Part model, mm, in its own coordinate system. Coordinates: 2 decimals unless noted, no trailing zeros. Order: outer loops, then holes, each group sorted by start corner. A loop starts at its lowest first (then second) coordinate and runs counter-clockwise, first axis right, second up.
from build123d import *

# Parameters (mm, degrees)
SKETCH019_W     = 73
SKETCH019_H     = 40
PAD006_DEPTH    = 5
SKETCH020_R     = 3
SKETCH020_R_2   = 1.75
POCKET011_DEPTH = 5
SKETCH021_R     = 3
POCKET012_DEPTH = 3.5
FILLET_R        = 1
POCKET014_DEPTH = 1


with BuildPart() as part:
    # Sketch019 → Pad006 (new body)
    with BuildSketch(Plane.XY):
        with Locations((36.5, 20)):
            Rectangle(SKETCH019_W, SKETCH019_H)
    extrude(amount=PAD006_DEPTH)

    # Sketch020 (on Face6 of Pad006) → Pocket011 (cut)
    with BuildSketch(Plane.XY.offset(5)):
        with Locations((14, 18.5)):
            Circle(SKETCH020_R)
        with Locations((59, 18.5)):
            Circle(SKETCH020_R)
        with Locations((36.5, 18.5)):
            Circle(SKETCH020_R)
        with Locations((9, 33.25)):
            Circle(SKETCH020_R_2)
        with Locations((64, 33.25)):
            Circle(SKETCH020_R_2)
        with Locations((64, 5.25)):
            Circle(SKETCH020_R_2)
        with Locations((9, 5.25)):
            Circle(SKETCH020_R_2)
    extrude(amount=-POCKET011_DEPTH, mode=Mode.SUBTRACT)

    # Sketch021 (on Face5 of Pocket011) → Pocket012 (cut)
    with BuildSketch(Plane.XY.offset(5)):
        with Locations((36.5, 18.5)):
            Circle(SKETCH021_R)
        with Locations((9, 5.25)):
            Circle(SKETCH021_R)
        with Locations((64, 33.25)):
            Circle(SKETCH021_R)
        with Locations((9, 33.25)):
            Circle(SKETCH021_R)
    extrude(amount=-POCKET012_DEPTH, mode=Mode.SUBTRACT)

    # Fillet
    fillet_edges = [part.edges().sort_by_distance(p)[0] for p in [
        (73, 20, 5),
        (36.5, 40, 5),
        (0, 20, 5),
        (36.5, 0, 5),
    ]]
    fillet(fillet_edges, radius=FILLET_R)

    # Sketch023 (on Face8 of Fillet) → Pocket014 (cut)
    with BuildSketch(Plane.XY.offset(5)):
        Polygon((36.5, 4), (38.5, 7), (34.5, 7), align=None)
    extrude(amount=-POCKET014_DEPTH, mode=Mode.SUBTRACT)


solid = part.part
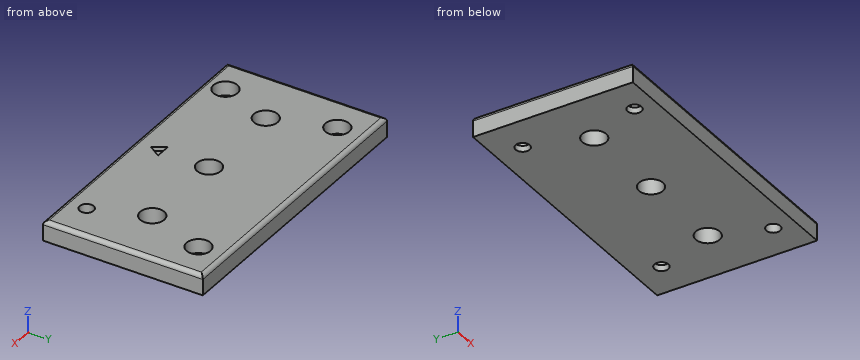
Q1. Cut at D-D on y = 5.25. Write the cut outline in (x, z), and give its area (3 significant figures).
Results list:
outline: (0, 0) - (7.25, 0) - (7.25, 1.5) - (6, 1.5) - (6, 5) - (1, 5) arc R1 ccw to (0, 4) - close; (10.75, 0) - (62.25, 0) - (62.25, 5) - (37.33, 5) - (37.33, 4) - (35.67, 4) - (35.67, 5) - (12, 5) - (12, 1.5) - (10.75, 1.5) - close; (65.75, 0) - (73, 0) - (73, 4) arc R1 ccw to (72, 5) - (65.75, 5) - close
area: 319 mm2
Q2. Cut at A-A on y = 33.25. Write the cut outline in (x, z), and give its area (3 significant figures).
Results list:
outline: (0, 0) - (7.25, 0) - (7.25, 1.5) - (6, 1.5) - (6, 5) - (1, 5) arc R1 ccw to (0, 4) - close; (10.75, 0) - (62.25, 0) - (62.25, 1.5) - (61, 1.5) - (61, 5) - (12, 5) - (12, 1.5) - (10.75, 1.5) - close; (65.75, 0) - (73, 0) - (73, 4) arc R1 ccw to (72, 5) - (67, 5) - (67, 1.5) - (65.75, 1.5) - close
area: 312 mm2
Q3. Wall check: line 1 along Y through (x, z) = (9, 2.55); line 2 along X through (y, z) = (21, 3.3); line 3 along Y through (x, z) = (64, 2.9). Give the ranges that are in metal, low to high.
Results list:
line 1: y = 0 to 2.25, 8.25 to 30.25, 36.25 to 40
line 2: x = 0 to 12.34, 15.66 to 34.84, 38.16 to 57.34, 60.66 to 73
line 3: y = 0 to 3.5, 7 to 30.25, 36.25 to 40
Q4. Pin check, flat tips, straight feed: pin 1 Ø3 at (x, y) = (10, 6) entering from +Z; pin 2 Ø9.5 at (x, y) = (64, 33.25) entering from +Z; pin 3 Ø5.5 at (x, y) = (59, 18.5) entering from -Z. Stop position of each tip, or through.
Results list:
pin 1: stops at z = 1.5
pin 2: stops at z = 5
pin 3: passes through
Q5. Cut at C-C on x = 14. Write the cut outline in (y, z).
Results list:
outline: (0, 0) - (15.5, 0) - (15.5, 5) - (1, 5) arc R1 ccw to (0, 4) - close; (21.5, 0) - (40, 0) - (40, 4) arc R1 ccw to (39, 5) - (21.5, 5) - close
Q6. Cut at B-B on y = 18.5. Write the cut outline in (x, z), and give its area (3 significant figures).
Results list:
outline: (0, 0) - (11, 0) - (11, 5) - (1, 5) arc R1 ccw to (0, 4) - close; (17, 0) - (33.5, 0) - (33.5, 5) - (17, 5) - close; (39.5, 0) - (56, 0) - (56, 5) - (39.5, 5) - close; (62, 0) - (73, 0) - (73, 4) arc R1 ccw to (72, 5) - (62, 5) - close
area: 275 mm2
